```python
from build123d import *

# Parameters (mm, degrees)
F0_W      = 30
F0_H      = 10
F1_DEPTH  = 120
F2_W      = 30
F2_H      = 10
F3_DEPTH  = 50
F4_W      = 10
F4_H      = 5
F5_DEPTH  = 30.001
F6_W      = 25
F6_H      = 10
F7_DEPTH  = 10.001
F8_W      = 20
F8_H      = 5
F9_DEPTH  = 45
F10_W     = 24
F10_H     = 110
F11_DEPTH = 12.5
F12_SIZE  = 5


with BuildPart() as f1:
    # F0 (on Front) → F1 (new body)
    with BuildSketch(Plane.XZ):
        Rectangle(F0_W, F0_H)
    extrude(amount=F1_DEPTH)

    # F2 (on face) → F3 (join)
    with BuildSketch(Plane.XZ.offset(120)):
        Rectangle(F2_W, F2_H)
    extrude(amount=F3_DEPTH)

    # F4 (on face) → F5 (cut, through all)
    with BuildSketch(Plane(origin=(-15, 0, 0), x_dir=(0, -1, 0), z_dir=(-1, 0, 0))):
        with Locations((160, 0)):
            Rectangle(F4_W, F4_H)
        with Locations((145, 0)):
            Rectangle(F4_W, F4_H)
        with Locations((130, 0)):
            Rectangle(F4_W, F4_H)
    extrude(amount=-F5_DEPTH, mode=Mode.SUBTRACT)

    # F6 (on face) → F7 (cut, through all)
    with BuildSketch(Plane.XY.offset(5)):
        with Locations((0, -160)):
            Rectangle(F6_W, F6_H)
        with Locations((0, -145)):
            Rectangle(F6_W, F6_H)
        with Locations((0, -130)):
            Rectangle(F6_W, F6_H)
    extrude(amount=-F7_DEPTH, mode=Mode.SUBTRACT)

    # F8 (on face) → F9 (cut)
    with BuildSketch(Plane.XZ.offset(170)):
        Rectangle(F8_W, F8_H)
    extrude(amount=-F9_DEPTH, mode=Mode.SUBTRACT)

    # F10 (on face) → F11 (join)
    with BuildSketch(Plane(origin=(0, 0, -5), x_dir=(1, 0, 0), z_dir=(0, 0, -1))):
        with Locations((0, 55)):
            Rectangle(F10_W, F10_H)
    extrude(amount=F11_DEPTH)

    # F12
    f12_edges = [f1.edges().sort_by_distance(p)[0] for p in [
        (0, -110, -17.5),
        (0, 0, -17.5),
    ]]
    chamfer(f12_edges, length=F12_SIZE)


solid = f1.part
```
Source: CAD feature listing. Evaluate the final solid. Frame: model axes, mm. A direction names the side the tool comes from. Round coordinates to 2 decimals unless told otherwise and drop trailing zeros. Write each loop counter-clockwise with the first axis right and the second up, starting at its lowest first coordinate (ties: lowest second). Pieces come first, ordered by that corner, then holes. Notation, with made-up numbers: M -27.5,43.25 L 23.5,43.25 A36 cw 23.5,77.25 Z; hole C -7.75,31 d8. An arc over 180 degrees is marked long. Answer as a JSON object with one key per item and string values. Group by question number.
(1) Ray query, line 1 (Y direction, x = 9, z = -4.5); line 2 (Y direction, x = -6.5, z = -6); line 3 (Z direction, x = -13, y = -16). Return the intervals inside material, ascending. Write a range as [from, to].
(2) Section query A-A on x = 6. State how many separate pieces and enclosed holes the cut face has, then the cut area to 4 significant figures.
(3) Reachability of faces 1 (the flat face through (12, -54, -11)), 2 (the flat face through (0, -153, 2.5)), 3 (the flat face through (0, -155, 3)) from +Z, -Z, +X, -X, +Y, -Y: full face, straight path, thin tool, end or side. Return the list, or none.
(4) Section query C-C on y = -23. Output: boundary loops of the cut face in (x, z).
(5) First-contact query: pin 1 (3 mm diameter, centred on x = 14.5, y = -159, fed in from -Z); pin 2 (3 mm diameter, centred on x = 7.5, z = 0.5, fed in from -Y). Flat tips, straight axial feed; report the tip coordinate or a pass-through.
(6) Section query B-B on z = 0. Output: boundary loops of the cut face in (x, y), then the cut area to 3 significant figures.
(7) Mould query, pull axis Z, two halves, no side actions, for faces 4 (the flat face through (0, -138, 2.5)), 5 (the flat face through (-0.2, -107.5, -15)), 6 (the flat face through (0, -138, -2.5)), 7 (the flat face through (15, -84, 0)). Classes: +Z half, -Z half, draft (parallel to the pull), parting line (faces both ways), or undercut.
(8) Section query D-D on z = -10.5. Output: boundary loops of the cut face in (x, y).
Computed values:
{
 "1": {"line 1": "[-170, -165], [-155, -150], [-140, -135], [-125, 0]", "line 2": "[-110, 0]", "line 3": "[-5, 5]"},
 "2": {"separate pieces": "7", "enclosed holes": "0", "area": "2,675 mm^2"},
 "3": {"face 1": "-Z, +X, +Y, -Y", "face 2": "-Y", "face 3": "none"},
 "4": {"outline": "M -15,-5 L -12,-5 L -12,-17.5 L 12,-17.5 L 12,-5 L 15,-5 L 15,5 L -15,5 Z"},
 "5": {"pin 1": "z = -5", "pin 2": "y = -125"},
 "6": {"outline": "M -15,-170 L -10,-170 L -10,-165 L -15,-165 Z; M -15,-155 L -10,-155 L -10,-150 L -15,-150 Z; M -15,-140 L -10,-140 L -10,-135 L -15,-135 Z; M -15,-125 L 15,-125 L 15,0 L -15,0 Z; M 10,-170 L 15,-170 L 15,-165 L 10,-165 Z; M 10,-155 L 15,-155 L 15,-150 L 10,-150 Z; M 10,-140 L 15,-140 L 15,-135 L 10,-135 Z", "area": "3,900 mm^2"},
 "7": {"face 4": "undercut", "face 5": "-Z half", "face 6": "undercut", "face 7": "draft"},
 "8": {"outline": "M -12,-110 L 12,-110 L 12,0 L -12,0 Z"}
}
